Design review of the part built by this model. Coordinates are the model's own, in mm. A direction names the side the tool comes from. Coordinates: 2 decimals unless noted, no trailing zeros. Loops run counter-clockwise (first coordinate to the right, second up) from the corner with the lowest first, then second, coordinate; pieces in that order, holes last. Notation, with made-up numbers: M -0.5,70.25 L 48.5,70.25 A29 ccw 48.5,105.25 Z; hole C 24,33 d9. An arc over 180 degrees is marked long. Put each result on its own line as item: value. Start each with the question number.
(1) Take a section at B-B, the plane y = 61. Give the boundary of the cut face in (x, z).
(2) Clearance check with flat-ended pins moving along their axes: pin 1 (3 mm diameter, centred on y = 33, z = 21.27, fed in from -X); pin 2 (5.5 mm diameter, centred on y = 61, z = 10.5, fed in from +X). State where each tip first meets the part, or that it passes through.
(3) For faces 1 (the flat face through (0, 47, 33.5)), 2 (the cylindrical face through (2.528, 64.794, 8.081)), list the 3-axis set-ups (+Z, -Z, +X, -X, +Y, -Y) from which the entire face can be reached by the end or side of a thin tool; tool diameter is ignored.
(4) Take a section at D-D, the plane x = -2. Give the boundary of the cut face in (y, z).
(5) Take a section at A-A, the plane z = 21.5. Give the boundary of the cut face in (x, y), then the cut area to 3 significant figures.
(6) Take a section at C-C, the plane z = 10.5. Give the boundary of the cut face in (x, y).
(7) The part is to be moulded in two halves that separate along Y. For faces 3 (the cylindrical face through (-2.528, 64.794, 12.919)), 4 (the flat face through (-0.5, 61, 10)), 5 (the flat face through (0, 47, 0)), 6 (the flat face through (0, 88.5, 17)), say which applies: +Y half, -Y half, draft (parallel to the pull), parting line (faces both ways), or undercut.
(8) For probe 1 along Y at (x, z) = (-2.55, 10.5); probe 2 along X at (y, z) = (61, 7.5); probe 3 along Z at (x, y) = (1.5, 64), list the stretches that pass through material, from the lowest coordinate up. Write a range as [from, to].
Autodesk Inventor part; units mm, degrees
ref_plane "Work Plane2" through (-89, -40.3889, 33.5) normal (0, 0, 1) x (1, 0, 0)
ref_plane "YZ Plane" through (0, 0, 0) normal (1, 0, 0) x (0, 1, 0)
ref_plane "XZ Plane" through (0, 0, 0) normal (0, 1, 0) x (-1, 0, 0)
ref_plane "Work Plane1" through (0, 0, 0) normal (0, 0, 1) x (1, 0, 0)
ref_plane "Work Plane2" through (-89, -40.3889, 33.5) normal (0, 0, 1) x (1, 0, 0)
sketch "Sketch1" plane through (0, 0, 0) normal (0, 0, 1) x (1, 0, 0)
  line L0 (23.5, 88.5) -> (-23.5, 88.5)
  line L1 (-23.5, 88.5) -> (-23.5, 36.5)
  line L2 (-26.5, 33.5) -> (-89, 33.5)
  line L3 (-89, 33.5) -> (-89, -72.5)
  line L4 (-89, -72.5) -> (-77, -72.5)
  line L5 (-74, -75.5) -> (-74, -93.5)
  line L6 (-74, -93.5) -> (74, -93.5)
  line L7 (74, -93.5) -> (74, -75.5)
  line L8 (77, -72.5) -> (89, -72.5)
  line L9 (89, -72.5) -> (89, 33.5)
  line L10 (89, 33.5) -> (26.5, 33.5)
  line L11 (23.5, 36.5) -> (23.5, 88.5)
  line L12 (-4.5, 81.5) -> (-4.5, 36.5)
  line L13 (-7.5, 33.5) -> (-13.5, 33.5)
  line L14 (-16.5, 36.5) -> (-16.5, 81.5)
  line L15 (-13.5, 84.5) -> (-7.5, 84.5)
  line L16 (16.5, 81.5) -> (16.5, 36.5)
  line L17 (13.5, 33.5) -> (7.5, 33.5)
  line L18 (4.5, 36.5) -> (4.5, 81.5)
  line L19 (7.5, 84.5) -> (13.5, 84.5)
  line L20 (-4.5, 88.5) -> (4.5, 88.5)
  line L21 (4.5, 88.5) -> (4.5, 3.75)
  line L22 (4.5, 3.75) -> (-4.5, 3.75)
  line L23 (-4.5, 3.75) -> (-4.5, 88.5)
  line L24 (-32.2, 4.75) -> (-59.9, 4.75)
  arc A0 (13.5, 33.5) -> (16.5, 36.5) centre (13.5, 36.5) ccw
  arc A1 (4.5, 36.5) -> (7.5, 33.5) centre (7.5, 36.5) ccw
  arc A2 (7.5, 84.5) -> (4.5, 81.5) centre (7.5, 81.5) ccw
  arc A3 (16.5, 81.5) -> (13.5, 84.5) centre (13.5, 81.5) ccw
  arc A4 (-4.5, 81.5) -> (-7.5, 84.5) centre (-7.5, 81.5) ccw
  arc A5 (-7.5, 33.5) -> (-4.5, 36.5) centre (-7.5, 36.5) ccw
  arc A6 (-16.5, 36.5) -> (-13.5, 33.5) centre (-13.5, 36.5) ccw
  arc A7 (-13.5, 84.5) -> (-16.5, 81.5) centre (-13.5, 81.5) ccw
  arc A8 (-26.5, 33.5) -> (-23.5, 36.5) centre (-26.5, 36.5) ccw
  arc A9 (-74, -75.5) -> (-77, -72.5) centre (-77, -75.5) ccw
  arc A10 (77, -72.5) -> (74, -75.5) centre (77, -75.5) ccw
  arc A11 (23.5, 36.5) -> (26.5, 33.5) centre (26.5, 36.5) ccw
  point P0 (0, 0)
  point P1 (-4.5, 81.5)
  point P2 (-4.5, 36.5)
  dimension "d0" = 1
extrude "Extrusion1" add sketch "Sketch1" along normal up to surface (33.5 mm away) contours L21 L18 L22 L23 L12 L0
sketch "Sketch2" plane through (4.5, 3.75, 0) normal (1, 0, 0) x (0, 0, -1)
  circle A0 centre (-21.2694, 29.2497) radius 2
  point P0 (0, -3.75)
extrude "Extrusion2" cut sketch "Sketch2" against normal blind 10
sketch "Sketch3" plane through (4.5, 3.75, 0) normal (1, 0, 0) x (0, 0, -1)
  circle A0 centre (-10.5, 57.25) radius 4.5
  point P0 (0, -3.75)
extrude "Extrusion3" cut sketch "Sketch3" against normal blind 4
sketch "Sketch4" plane through (-4.5, 3.75, 0) normal (-1, 0, 0) x (0, 0, 1)
  circle A0 centre (10.5, 57.25) radius 4.5
  point P0 (0, -3.75)
extrude "Extrusion4" cut sketch "Sketch4" against normal blind 4
properties part number "middle_gear_holder"
Computed values:
1. outline: M -4.5,0 L 4.5,0 L 4.5,6 L 0.5,6 L 0.5,15 L 4.5,15 L 4.5,33.5 L -4.5,33.5 L -4.5,15 L -0.5,15 L -0.5,6 L -4.5,6 Z
2. pin 1: passes through
2. pin 2: stops at x = 0.5
3. face 1: +Z, +X, -X, +Y, -Y
3. face 2: +X
4. outline: M 3.75,0 L 88.5,0 L 88.5,33.5 L 3.75,33.5 Z; hole C 33,21.27 d4; hole C 61,10.5 d9
5. outline: M -4.5,3.75 L 4.5,3.75 L 4.5,31.01 L -4.5,31.01 Z; M -4.5,34.99 L 4.5,34.99 L 4.5,88.5 L -4.5,88.5 Z
5. area: 727 mm^2
6. outline: M -4.5,3.75 L 4.5,3.75 L 4.5,56.5 L 0.5,56.5 L 0.5,65.5 L 4.5,65.5 L 4.5,88.5 L -4.5,88.5 L -4.5,65.5 L -0.5,65.5 L -0.5,56.5 L -4.5,56.5 Z
7. face 3: undercut
7. face 4: undercut
7. face 5: draft
7. face 6: +Y half
8. probe 1: y = [3.75, 56.5], [65.5, 88.5]
8. probe 2: x = [-0.5, 0.5]
8. probe 3: z = [0, 7.15], [13.85, 33.5]
